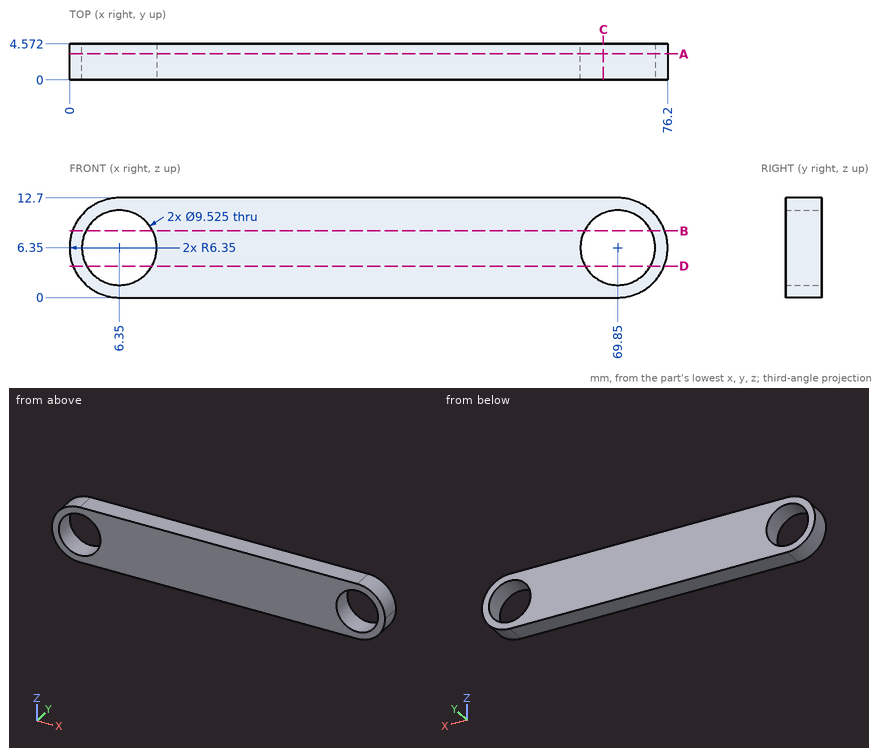
Drawing for the job (mm, zero at the part's lowest x, y, z). Round coordinates to 2 decimals unless told otherwise and drop trailing zeros. Loops run counter-clockwise (first coordinate to the right, second up) from the corner with the lowest first, then second, coordinate; pieces in that order, holes last. Notation, with made-up numbers: (-9, 79) - (18, 79) arc R26 ccw to (18, 96) - close; hole circle Ø7 at (81.25, 89). An arc over 180 degrees is marked (long way). Return JSON: item names as keys, results as strings. Group by question number.
Q1. Band-saw the part on D-D on z = 4. Give the cut face in (x, y), plus the area to 3 significant figures.
Q2. Band-saw the part on B-B on z = 8.5. Give the cut face in (x, y).
Q3. Flat gauge pins, fed straight in: pin 1 Ø5.5 at (x, z) = (6.35, 6.35) entering from -Y (3 decimals); pin 2 Ø1 at (y, z) = (2, 5) entering from +X. Where does each tip first touch, or does it go through?
Q4. Drill centre lines: line 1 along X through (y, z) = (0.6, 6.25); line 2 along X through (y, z) = (1.15, 5); line 3 along Z through (x, y) = (69.85, 3.1). Where is each one in solid material? Low to high. Write a range as [from, to].
Q5. Band-saw the part on C-C on x = 68. Give the cut face in (y, z), plus the area to 3 significant figures.
Q6. Band-saw the part on A-A on y = 3.3. Give the number of separate pieces and of enclosed holes in the cut face, plus the area to 3 significant figures.
Solutions:
{
 "1": {"outline": "(0.45, 0) - (2.21, 0) - (2.21, 4.57) - (0.45, 4.57) - close; (10.49, 0) - (65.71, 0) - (65.71, 4.57) - (10.49, 4.57) - close; (73.99, 0) - (75.75, 0) - (75.75, 4.57) - (73.99, 4.57) - close", "area": "269 mm^2"},
 "2": {"outline": "(0.38, 0) - (2.1, 0) - (2.1, 4.57) - (0.38, 4.57) - close; (10.6, 0) - (65.6, 0) - (65.6, 4.57) - (10.6, 4.57) - close; (74.1, 0) - (75.82, 0) - (75.82, 4.57) - (74.1, 4.57) - close"},
 "3": {"pin 1": "passes through", "pin 2": "stops at x = 76.14"},
 "4": {"line 1": "x = [0, 1.59], [11.11, 65.09], [74.61, 76.2]", "line 2": "x = [0.15, 1.78], [10.92, 65.28], [74.42, 76.05]", "line 3": "z = [0, 1.59], [11.11, 12.7]"},
 "5": {"outline": "(0, 0) - (4.57, 0) - (4.57, 1.96) - (0, 1.96) - close; (0, 10.74) - (4.57, 10.74) - (4.57, 12.7) - (0, 12.7) - close", "area": "17.9 mm^2"},
 "6": {"separate pieces": "1", "enclosed holes": "2", "area": "791 mm^2"}
}
